For this review, take the finished solid that the model builds, in its own axes (mm). Coordinates: 2 decimals unless noted, no trailing zeros. Loops run counter-clockwise (first coordinate to the right, second up) from the corner with the lowest first, then second, coordinate; pieces in that order, holes last. Notation, with made-up numbers: M -38,18.25 L -21,18.25 A17 ccw -21,47.25 Z; hole C -26,37 d3. An arc over 180 degrees is marked long. Use one line per item in the form item = value.
```python
from build123d import *

# Parameters (mm, degrees)
SKETCH2_W           = 140
SKETCH2_H           = 2700
SKETCH2_R           = 50
BOSS_EXTRUDE1_DEPTH = 50


with BuildPart() as part:
    # Sketch2 → Boss-Extrude1 (new body)
    with BuildSketch(Plane.ZX):
        with Locations((22932.944645813, -11431.030459334)):
            Rectangle(SKETCH2_W, SKETCH2_H)
        with Locations((22932.944645813, -12681.030459334)):
            Circle(SKETCH2_R, mode=Mode.SUBTRACT)
        with Locations((22932.944645813, -11431.030459334)):
            Circle(SKETCH2_R, mode=Mode.SUBTRACT)
        with Locations((22932.944645813, -10181.030459334)):
            Circle(SKETCH2_R, mode=Mode.SUBTRACT)
    extrude(amount=BOSS_EXTRUDE1_DEPTH)


solid = part.part
```
1. Wall thickness on line 1 along X through (y, z) = (40, 22935); line 2 along X through (y, z) = (32, 22887); line 3 along Z through (x, y) = (-10216, 5.5): over which ranges is each line inside the solid? List them lowest first. Write a range as from..to.
Computed values:
line_1 = -12781.03..-12730.99, -12631.07..-11480.99, -11381.07..-10230.99, -10131.07..-10081.03
line_2 = -12781.03..-12700.76, -12661.31..-11450.76, -11411.31..-10200.76, -10161.31..-10081.03
line_3 = 22862.94..22897.21, 22968.68..23002.94
2. Draft analysis for pull direction X (two halves, no side actions). For faces 1 (the face through (-11450, 25, 23002.945)), 2 (the face through (-10081.03, 25, 22932)), 3 (the face through (-12678.832, 24.65, 22882.993)), 4 (the face through (-12781.03, 25, 22932)), state which applies: +X half, -X half, draft (parallel to the pull), parting line (faces both ways), or undercut.
Computed values:
face_1 = draft
face_2 = +X half
face_3 = undercut
face_4 = -X half
3. Consider section A-A on z = 22943. Write out the cut boundary in (x, y).
Computed values:
outline = M -12781.03,0 L -12730.01,0 L -12730.01,50 L -12781.03,50 Z; M -12632.05,0 L -11480.01,0 L -11480.01,50 L -12632.05,50 Z; M -11382.05,0 L -10230.01,0 L -10230.01,50 L -11382.05,50 Z; M -10132.05,0 L -10081.03,0 L -10081.03,50 L -10132.05,50 Z
4. Consider section B-B on y = 29.5. Write out the cut boundary in (x, z).
Computed values:
outline = M -12781.03,22862.94 L -10081.03,22862.94 L -10081.03,23002.94 L -12781.03,23002.94 Z; hole C -12681.03,22932.94 d100; hole C -11431.03,22932.94 d100; hole C -10181.03,22932.94 d100
